from build123d import *

# Parameters (mm, degrees)
F5_W     = 42.267536
F5_H     = 10.794579
F6_DEPTH = 30
F7_R     = 1.875564
F8_DEPTH = 25


with BuildPart() as f1:
    # F0 (on Front) → F1 (revolve)
    with BuildSketch(Plane.XZ):
        with BuildLine():
            Line((0, 0), (0, -17.5))
            ThreePointArc((0, -17.5), (17.5, 0), (0, 17.5))
            Line((0, 17.5), (0, 0))
        make_face()
    revolve(axis=Axis((0, 0, -8.75), (0, 0, -1)))


with BuildPart() as f3:
    # F2 (on Front) → F3 (revolve)
    with BuildSketch(Plane.XZ):
        with BuildLine():
            Line((0, 15), (0, -15))
            ThreePointArc((0, -15), (15, 0), (0, 15))
        make_face()
    revolve(axis=Axis((0, 0, 8.75), (0, 0, 1)))


with BuildPart() as f1_1:
    add(f1.part)

    # F4: cut F3
    add(f3.part, mode=Mode.SUBTRACT)

    # F5 (on Front) → F6 (cut, symmetric)
    with BuildSketch(Plane.XZ):
        with Locations((1.34061, -15.593321)):
            Rectangle(F5_W, F5_H)
    extrude(amount=F6_DEPTH, both=True, mode=Mode.SUBTRACT)

    # F7 (on Top) → F8 (cut)
    with BuildSketch(Plane.XY):
        Circle(F7_R)
    extrude(amount=F8_DEPTH, mode=Mode.SUBTRACT)


solid = f1_1.part
Could you check a few things on this model? Use its own coordinates, in mm. Give positions to 0.01 mm unless a question says otherwise; leave off trailing zeros. Loops run counter-clockwise (first coordinate to the right, second up) from the corner with the lowest first, then second, coordinate; pieces in that order, holes last. Notation, with made-up numbers: M 73,-24 L 122,-24 A27 cw 122,5 Z; hole C 7,49.5 d3. An arc over 180 degrees is marked long. Answer as a JSON object with one key per item and string values.
Q1. If we mould it in two halves opening along Y, with no side actions, what happens to faces 1 (the flat face through (4.1, 10.5, -10.196)), 2 (the cylindrical face through (-1.38, 1.27, 16.12))? For each: pulls with the +Y half, pulls with the -Y half, needs draft (parallel to the pull), parting line crosses it, or undercut.
Values found:
{"face 1": "needs draft", "face 2": "undercut"}
Q2. Suppose I cut it at C-C, the plane x = 13.5. List the corners of the cut face in (y, z) for me, plus the area to 3 significant figures.
Values found:
{"outline": "M -4.48,-10.2 L 4.48,-10.2 A11.14 ccw long Z; hole C 0,0 d13.08", "area": "250 mm²"}
Q3. Suppose I cut it at A-A, the plane x = 0. List the corners of the cut face in (y, z) for me, plus the area to 3 significant figures.
Values found:
{"outline": "M -14.22,-10.2 L -11,-10.2 A15 cw -1.88,14.88 L -1.88,17.4 A17.5 ccw Z; M 1.88,14.88 A15 cw 11,-10.2 L 14.22,-10.2 A17.5 ccw 1.88,17.4 Z", "area": "173 mm²"}
Q4. If I drill on probe 1 along X at (y, z) = (-5, 4.5); probe 2 along Z at (x, y) = (-13, 2); probe 3 along X at (y, z) = (-4, 3.5), over which ranges is the centre line in solid material (lowest first)? Write a range as [from, to].
Values found:
{"probe 1": "x = [-16.16, -13.41], [13.41, 16.16]", "probe 2": "z = [-10.2, -7.21], [7.21, 11.54]", "probe 3": "x = [-16.67, -14.03], [14.03, 16.67]"}
Q5. Suppose I cut it at D-D, the plane z = 3.75. List the corners of the cut face in (x, y) for me, plus the area to 3 significant figures.
Values found:
{"outline": "C 0,0 d34.19; hole C 0,0 d29.05", "area": "255 mm²"}
Q6. For P1, Ø2, axis at x = -7, z = 11, coming from the +Y side; P2, Ø6, axis at x = -8.5, y = -9.5, coming from the +Z side; P3, Ø10, axis at y = -13.5, z = -6.5, coming from the +X side; P4, Ø2.5, axis at x = 0, y = 0, coming from the -Z side, each with a flat end and sliding along its axis, tell me the tip position at first contact or that it passes through.
Values found:
{"P1": "stops at y = 12.7", "P2": "stops at z = 14.53", "P3": "stops at x = 14.37", "P4": "passes through"}
